```python
from build123d import *

# Parameters (mm, degrees)
CROQUIS1_R              = 1.5
CROQUIS1_W              = 25
CROQUIS1_H              = 72
CROQUIS1_W_2            = 3.5
CROQUIS1_H_2            = 40.5
SALIENTE_EXTRUIR1_DEPTH = 3


with BuildPart() as part:
    # Croquis1 → Saliente-Extruir1 (new body)
    with BuildSketch(Plane.XY):
        Polygon((-75, -75), (-75, -65), (-72, -65), (-72, -55), (-75, -55), (-75, -45), (-72, -45), (-72, -35), (-75, -35), (-75, -25), (-72, -25), (-72, -15), (-75, -15), (-75, -5), (-72, -5), (-72, 5), (-75, 5), (-75, 15), (-72, 15), (-72, 25), (-75, 25), (-75, 35), (-72, 35), (-72, 45), (-75, 45), (-75, 55), (-72, 55), (-72, 65), (-75, 65), (-75, 75), (-65, 75), (-65, 72), (-55, 72), (-55, 75), (-45, 75), (-45, 72), (-35, 72), (-35, 75), (-25, 75), (-25, 72), (-15, 72), (-15, 75), (-5, 75), (-5, 72), (5, 72), (5, 75), (15, 75), (15, 72), (25, 72), (25, 75), (35, 75), (35, 72), (45, 72), (45, 75), (55, 75), (55, 72), (65, 72), (65, 75), (75, 75), (75, 65), (72, 65), (72, 55), (75, 55), (75, 45), (72, 45), (72, 35), (75, 35), (75, 25), (72, 25), (72, 15), (75, 15), (75, 5), (72, 5), (72, -5), (75, -5), (75, -15), (72, -15), (72, -25), (75, -25), (75, -35), (72, -35), (72, -45), (75, -45), (75, -55), (72, -55), (72, -65), (75, -65), (75, -75), (65, -75), (65, -72), (55, -72), (55, -75), (45, -75), (45, -72), (35, -72), (35, -75), (25, -75), (25, -72), (15, -72), (15, -75), (5, -75), (5, -72), (-5, -72), (-5, -75), (-15, -75), (-15, -72), (-25, -72), (-25, -75), (-35, -75), (-35, -72), (-45, -72), (-45, -75), (-55, -75), (-55, -72), (-65, -72), (-65, -75), align=None)
        with Locations((20, 37.5)):
            Circle(CROQUIS1_R, mode=Mode.SUBTRACT)
        with Locations(Location((51, 37.5, 0), (0, 0, 180))):
            Circle(CROQUIS1_R, mode=Mode.SUBTRACT)
        with Locations((51, -37.5)):
            Circle(CROQUIS1_R, mode=Mode.SUBTRACT)
        with Locations(Location((20, -37.5, 0), (0, 0, 180))):
            Circle(CROQUIS1_R, mode=Mode.SUBTRACT)
        with Locations((34.5, 0)):
            Rectangle(CROQUIS1_W, CROQUIS1_H, mode=Mode.SUBTRACT)
        with Locations((51.25, 13.75)):
            Rectangle(CROQUIS1_W_2, CROQUIS1_H_2, mode=Mode.SUBTRACT)
    extrude(amount=SALIENTE_EXTRUIR1_DEPTH)


solid = part.part
```
Work out the finished part from the listing and answer in its coordinate system (mm). Give positions to 0.01 mm unless a question says otherwise; leave off trailing zeros. Loops run counter-clockwise (first coordinate to the right, second up) from the corner with the lowest first, then second, coordinate; pieces in that order, holes last. Notation, with made-up numbers: (48, 34.5) -> (70, 34.5) arc R34 cw to (70, 65.5) -> close; hole circle Ø6 at (-14, -6.75). An arc over 180 degrees is marked (long way). Write item = value, one per line. Start each with the question number.
(1) Find section A-A on y = -19. Give the vertices of the cut face in (x, z), and give its area (3 significant figures).
(2) Find the intervals of material crossed by probe 1 along X at (y, z) = (23, 2.4); probe 2 along Y at (x, z) = (51, 1.5); probe 3 along Y at (x, z) = (20, 1.5), in increasing order. Write a range as from..to.
(3) Find section C-C on x = -40. Give the vertices of the cut face in (y, z).
(4) Find section B-B on z = 2.1. Give the number of separate pieces and of enclosed holes in the cut face, and give its area (3 significant figures).
(5) Given pin 1 Ø1 at (x, y) = (-26.5, 33.5) entering from -Z; pin 2 Ø0.9 at (y, z) = (60, 2) entering from +X; pin 3 Ø1.5 at (x, z) = (-42, 0.5) entering from +Y, each flat-ended and moving along its own axis, determine where each tip first touches the part or whether it passes through.
From the geometry:
q1.outline = (-72, 0) -> (22, 0) -> (22, 3) -> (-72, 3) -> close; (47, 0) -> (72, 0) -> (72, 3) -> (47, 3) -> close
q1.area = 357 mm^2
q2.probe_1 = -72..22, 47..49.5, 53..72
q2.probe_2 = -75..-39, -36..-6.5, 34..36, 39..75
q2.probe_3 = -72..-39, -36..36, 39..72
q3.outline = (-72, 0) -> (72, 0) -> (72, 3) -> (-72, 3) -> close
q4.separate_pieces = 1
q4.enclosed_holes = 6
q4.area = 19,700 mm^2
q5.pin_1 = 0
q5.pin_2 = 72
q5.pin_3 = 72
